The listing builds one solid part. Answer for the finished solid, in the listing's coordinates (mm). Coordinates: 2 decimals unless noted, no trailing zeros. Order: outer loops, then holes, each group sorted by start corner. A loop starts at its lowest first (then second) coordinate and runs counter-clockwise, first axis right, second up. Notation, with made-up numbers: (45, 39.25) -> (51, 39.25) arc R14 ccw to (51, 49.25) -> close; hole circle Ø10 at (-15.75, -18.5). An arc over 180 degrees is marked (long way). Return JSON: item names as keys, results as strings.
from build123d import *

# Parameters (mm, degrees)
F0_R     = 75
F0_R_2   = 26.5
F1_DEPTH = 2
F2_R     = 48.5
F2_R_2   = 26.5
F3_DEPTH = 50
F4_R     = 1.75
F5_DEPTH = 2.001


with BuildPart() as f1:
    # F0 (on Top) → F1 (new body)
    with BuildSketch(Plane.XY):
        Circle(F0_R)
        with BuildLine():
            Line((-43.513595, -11.470269), (-28.389388, -8.018268))
            ThreePointArc((-28.389388, -8.018268), (-23.064029, -18.392949), (-14.134466, -25.893375))
            Line((-14.134466, -25.893375), (-20.865371, -39.870243))
            ThreePointArc((-20.865371, -39.870243), (-35.182417, -28.057041), (-43.513595, -11.470269))
        make_face(mode=Mode.SUBTRACT)
        with BuildLine():
            Line((-18.162465, -41.171894), (-11.43156, -27.195026))
            ThreePointArc((-11.43156, -27.195026), (0, -29.5), (11.43156, -27.195026))
            Line((11.43156, -27.195026), (18.162465, -41.171894))
            ThreePointArc((18.162465, -41.171894), (0, -45), (-18.162465, -41.171894))
        make_face(mode=Mode.SUBTRACT)
        with BuildLine():
            Line((20.865371, -39.870243), (14.134466, -25.893375))
            ThreePointArc((14.134466, -25.893375), (23.064029, -18.392949), (28.389388, -8.018268))
            Line((28.389388, -8.018268), (43.513595, -11.470269))
            ThreePointArc((43.513595, -11.470269), (35.182417, -28.057041), (20.865371, -39.870243))
        make_face(mode=Mode.SUBTRACT)
        with BuildLine():
            Line((-36.0981, 26.868702), (-23.969429, 17.196409))
            ThreePointArc((-23.969429, 17.196409), (-28.760373, 6.564368), (-29.056951, -5.093484))
            Line((-29.056951, -5.093484), (-44.181157, -8.545486))
            ThreePointArc((-44.181157, -8.545486), (-43.871756, 10.013442), (-36.0981, 26.868702))
        make_face(mode=Mode.SUBTRACT)
        with BuildLine():
            Line((-1.5, 44.974993), (-1.5, 29.46184))
            ThreePointArc((-1.5, 29.46184), (-12.79957, 26.578582), (-22.098959, 19.541904))
            Line((-22.098959, 19.541904), (-34.227631, 29.214197))
            ThreePointArc((-34.227631, 29.214197), (-19.524768, 40.543599), (-1.5, 44.974993))
        make_face(mode=Mode.SUBTRACT)
        Circle(F0_R_2, mode=Mode.SUBTRACT)
        with BuildLine():
            Line((44.181157, -8.545486), (29.056951, -5.093484))
            ThreePointArc((29.056951, -5.093484), (28.760373, 6.564368), (23.969429, 17.196409))
            Line((23.969429, 17.196409), (36.0981, 26.868702))
            ThreePointArc((36.0981, 26.868702), (43.871756, 10.013442), (44.181157, -8.545486))
        make_face(mode=Mode.SUBTRACT)
        with BuildLine():
            ThreePointArc((22.098959, 19.541904), (12.79957, 26.578582), (1.5, 29.46184))
            Line((1.5, 29.46184), (1.5, 44.974993))
            ThreePointArc((1.5, 44.974993), (19.524768, 40.543599), (34.227631, 29.214197))
            Line((34.227631, 29.214197), (22.098959, 19.541904))
        make_face(mode=Mode.SUBTRACT)
    extrude(amount=F1_DEPTH)

    # F2 (on face) → F3 (join)
    with BuildSketch(Plane.XY.offset(2)):
        Circle(F2_R)
        with BuildLine():
            Line((-14.134466, -25.893375), (-20.865371, -39.870243))
            ThreePointArc((-20.865371, -39.870243), (-35.182417, -28.057041), (-43.513595, -11.470269))
            Line((-43.513595, -11.470269), (-28.389388, -8.018268))
            ThreePointArc((-28.389388, -8.018268), (-23.064029, -18.392949), (-14.134466, -25.893375))
        make_face(mode=Mode.SUBTRACT)
        with BuildLine():
            ThreePointArc((18.162465, -41.171894), (0, -45), (-18.162465, -41.171894))
            Line((-18.162465, -41.171894), (-11.43156, -27.195026))
            ThreePointArc((-11.43156, -27.195026), (0, -29.5), (11.43156, -27.195026))
            Line((11.43156, -27.195026), (18.162465, -41.171894))
        make_face(mode=Mode.SUBTRACT)
        with BuildLine():
            ThreePointArc((43.513595, -11.470269), (35.182417, -28.057041), (20.865371, -39.870243))
            Line((20.865371, -39.870243), (14.134466, -25.893375))
            ThreePointArc((14.134466, -25.893375), (23.064029, -18.392949), (28.389388, -8.018268))
            Line((28.389388, -8.018268), (43.513595, -11.470269))
        make_face(mode=Mode.SUBTRACT)
        with BuildLine():
            Line((-29.056951, -5.093484), (-44.181157, -8.545486))
            ThreePointArc((-44.181157, -8.545486), (-43.871756, 10.013442), (-36.0981, 26.868702))
            Line((-36.0981, 26.868702), (-23.969429, 17.196409))
            ThreePointArc((-23.969429, 17.196409), (-28.760373, 6.564368), (-29.056951, -5.093484))
        make_face(mode=Mode.SUBTRACT)
        with BuildLine():
            Line((-22.098959, 19.541904), (-34.227631, 29.214197))
            ThreePointArc((-34.227631, 29.214197), (-19.524768, 40.543599), (-1.5, 44.974993))
            Line((-1.5, 44.974993), (-1.5, 29.46184))
            ThreePointArc((-1.5, 29.46184), (-12.79957, 26.578582), (-22.098959, 19.541904))
        make_face(mode=Mode.SUBTRACT)
        Circle(F2_R_2, mode=Mode.SUBTRACT)
        with BuildLine():
            ThreePointArc((36.0981, 26.868702), (43.871756, 10.013442), (44.181157, -8.545486))
            Line((44.181157, -8.545486), (29.056951, -5.093484))
            ThreePointArc((29.056951, -5.093484), (28.760373, 6.564368), (23.969429, 17.196409))
            Line((23.969429, 17.196409), (36.0981, 26.868702))
        make_face(mode=Mode.SUBTRACT)
        with BuildLine():
            Line((1.5, 29.46184), (1.5, 44.974993))
            ThreePointArc((1.5, 44.974993), (19.524768, 40.543599), (34.227631, 29.214197))
            Line((34.227631, 29.214197), (22.098959, 19.541904))
            ThreePointArc((22.098959, 19.541904), (12.79957, 26.578582), (1.5, 29.46184))
        make_face(mode=Mode.SUBTRACT)
    extrude(amount=F3_DEPTH)

    # F4 (on face) → F5 (cut, through all)
    with BuildSketch(Plane.XY.offset(2)):
        with Locations((-4.894284, 71.231538)):
            Circle(F4_R)
        with Locations((4.654726, 71.307522)):
            Circle(F4_R)
    extrude(amount=-F5_DEPTH, mode=Mode.SUBTRACT)


solid = f1.part
1. The part is cut by section D-D on x = -40. Give the vertices of the cut face in (y, z), and give its area (3 significant figures).
Answer block:
{"outline": "(-63.44, 0) -> (-20.62, 0) -> (-20.62, 52) -> (-27.43, 52) -> (-27.43, 2) -> (-63.44, 2) -> close; (-10.67, 0) -> (-7.59, 0) -> (-7.59, 52) -> (-10.67, 52) -> close; (20.62, 0) -> (63.44, 0) -> (63.44, 2) -> (27.43, 2) -> (27.43, 52) -> (20.62, 52) -> close", "area": "1,010 mm2"}
2. Each of these flat-tipped pins is pushed along its axis until it touches: pin 1 Ø17 at (y, z) = (39.5, 38) entering from +X; pin 2 Ø5 at (y, z) = (-37.5, 6.5) entering from -X; pin 3 Ø3 at (y, z) = (-20, 7) entering from -X. Where does it stop, or does it pass through?
Answer block:
{"pin 1": "stops at x = 37.3", "pin 2": "stops at x = -33.57", "pin 3": "stops at x = -44.83"}
3. The part is cut by section A-A on y = 0. Give the vertices of the cut face in (x, z), and give its area (3 significant figures).
Answer block:
{"outline": "(-75, 0) -> (-45, 0) -> (-45, 52) -> (-48.5, 52) -> (-48.5, 2) -> (-75, 2) -> close; (-29.5, 0) -> (-26.5, 0) -> (-26.5, 52) -> (-29.5, 52) -> close; (26.5, 0) -> (29.5, 0) -> (29.5, 52) -> (26.5, 52) -> close; (45, 0) -> (75, 0) -> (75, 2) -> (48.5, 2) -> (48.5, 52) -> (45, 52) -> close", "area": "782 mm2"}
4. The part is cut by section B-B on z = 28.5. Give the number of separate pieces and of enclosed holes in the cut face, and give its area (3 significant figures).
Answer block:
{"separate pieces": "1", "enclosed holes": "8", "area": "1,880 mm2"}
5. The part is cut by section C-C on x = 16. Give the vertices of the cut face in (y, z), and give its area (3 significant figures).
Answer block:
{"outline": "(-73.27, 0) -> (-42.06, 0) -> (-42.06, 52) -> (-45.78, 52) -> (-45.78, 2) -> (-73.27, 2) -> close; (-36.68, 0) -> (-29.77, 0) -> (-29.77, 52) -> (-36.68, 52) -> close; (-24.78, 0) -> (-21.12, 0) -> (-21.12, 52) -> (-24.78, 52) -> close; (21.12, 0) -> (24.78, 0) -> (24.78, 52) -> (21.12, 52) -> close; (42.06, 0) -> (73.27, 0) -> (73.27, 2) -> (45.78, 2) -> (45.78, 52) -> (42.06, 52) -> close", "area": "1,240 mm2"}
6. Consider line 1 (Y direction, x = -1, z = 4.5); line 2 (X direction, y = 21, z = 26); line 3 (Y direction, x = -22.5, z = 35). Determine where each line is inside the solid, lowest interval first. Write a range as from..to.
Answer block:
{"line 1": "y = -48.49..-44.99, -29.48..-26.48, 26.48..48.49", "line 2": "x = -43.72..-39.8, -28.74..-23.93, -20.72..-16.16, 16.16..20.72, 23.93..28.74, 39.8..43.72", "line 3": "y = -42.97..-38.97, -19.08..-14, 14..19.86, 38.97..42.97"}
